Part model, mm, in its own coordinate system. A direction names the side the tool comes from. Round coordinates to 2 decimals unless told otherwise and drop trailing zeros. Loops run counter-clockwise (first coordinate to the right, second up) from the corner with the lowest first, then second, coordinate; pieces in that order, holes last.
Autodesk Inventor part; units mm, degrees
ref_plane "YZ Plane" through (0, 0, 0) normal (1, 0, 0) x (0, 1, 0)
ref_plane "XZ Plane" through (0, 0, 0) normal (0, 1, 0) x (-1, 0, 0)
ref_plane "XY Plane" through (0, 0, 0) normal (0, 0, 1) x (1, 0, 0)
sketch "Sketch1" plane through (0, 0, 0) normal (0, 1, 0) x (-1, 0, 0)
  line L0 (0.0381, -21.3061) -> (0.0381, -411.3061)
  line L1 (0.0381, -411.3061) -> (21.2513, -432.5193)
  line L2 (0.0381, -411.3061) -> (30.0381, -411.3061) construction
  line L3 (21.2513, -432.5193) -> (221.2513, -432.5193)
  line L4 (221.2513, -432.5193) -> (270.7487, -383.0218)
  line L5 (270.7487, -383.0218) -> (390.7487, -383.0218)
  line L6 (390.7487, -383.0218) -> (447.3173, -439.5904)
  line L7 (447.3173, -439.5904) -> (487.3173, -439.5904)
  line L8 (487.3173, -439.5904) -> (543.8858, -383.0218)
  line L9 (-53.2718, -216.3061) -> (592.6367, -216.3061) construction
  line L10 (0.0381, -21.3061) -> (21.2513, -0.0929)
  line L11 (21.2513, -0.0929) -> (221.2513, -0.0929)
  line L12 (221.2513, -0.0929) -> (270.7487, -49.5904)
  line L13 (270.7487, -49.5904) -> (390.7487, -49.5904)
  line L14 (390.7487, -49.5904) -> (447.3173, 6.9782)
  line L15 (447.3173, 6.9782) -> (487.3173, 6.9782)
  line L16 (487.3173, 6.9782) -> (543.8858, -49.5904)
  line L17 (543.8858, -383.0218) -> (543.8858, -49.5904)
  point P0 (0, 0)
  dimension "d0" = 390
  dimension "d1" = 30
  dimension "d2" = 45
  dimension "d3" = 70
  dimension "d4" = 135
  dimension "d5" = 200
  dimension "d6" = 120
  dimension "d7" = 80
  dimension "d8" = 135
  dimension "d9" = 226.066
  dimension "d10" = 21.2132
  dimension "d11" = 40
  dimension "d12" = 80
  dimension "d15" = 543.8478
extrude "Extrusion1" add sketch "Sketch1" along normal blind 200
sketch "Sketch2" plane through (-221.2513, 0, -0.0929) normal (0, 0, 1) x (1, 0, 0)
  line L0 (200, 0) -> (200, 200) construction
  line L1 (200, 50) -> (-356.3945, 50) construction
  line L2 (0, 0) -> (200, 0) construction
  line L3 (91.2132, 236.2215) -> (91.2132, -57.6692) construction
  line L4 (221.2132, 0) -> (221.2132, 200) construction
  point P0 (221.2513, 0)
  dimension "d18" = 50
  dimension "d19" = 130
sketch "Sketch3" plane through (-221.2513, 0, -0.0929) normal (0, 0, 1) x (1, 0, 0)
  line L0 (91.2132, 236.2215) -> (91.2132, -57.6692) construction
  line L1 (200, 50) -> (-356.3945, 50) construction
  circle A0 centre (91.2132, 50) radius 25
  point P0 (221.2513, 0)
  dimension "d20" = 50
properties part number "Frame"
1) Slice it at C-C, the plane x = -368. Give the cut face in (y, z).
Values:
outline: (0, -383.02) - (200, -383.02) - (200, -49.59) - (0, -49.59) - close
2) Mould opens along X. For faces 5 (the face through (-10.496, 98.6, -421.764)), 6 (the face through (-467, 99, -439.59)), 7 (the face through (-418.64, 98.6, -21.7)) say: released by +X, released by -X, zero draft, split by the parting line, or undercut.
Values:
face 5: released by +X
face 6: zero draft
face 7: undercut
3) Drop flat-ended pins along their axis: pin 1 Ø3 at (x, y) = (-288.5, 102.5) entering from +Z; pin 2 Ø10 at (x, y) = (-152.5, 49) entering from -Z; pin 3 Ø1 at (x, y) = (-249.5, 80) entering from -Z. Give the stop position or say it passes through.
Values:
pin 1: stops at z = -49.59
pin 2: stops at z = -432.52
pin 3: stops at z = -404.77
4) Tool access for faces 1 (the face through (-120, 99, -432.519)), 2 (the face through (-330, 99, -383.022)), 3 (the face through (-245.654, 98.6, -24.495)), 4 (the face through (-120, 99, -0.093)): list every direction of +Z, -Z, +X, -X, +Y, -Y with a clear straight run to the whole face (end or side of a thin tool).
Values:
face 1: -Z, +X, +Y, -Y
face 2: -Z, +Y, -Y
face 3: +Z, +Y, -Y
face 4: +Z, +X, +Y, -Y
5) Wall check: line 1 along Z through (x, y) = (-213.5, 108); line 2 along X through (y, z) = (144.5, -412.5); line 3 along Z through (x, y) = (-360, 170). Give the ranges that are in metal, low to high.
Values:
line 1: z = -432.52 to -0.09
line 2: x = -514.41 to -420.23, -241.27 to -1.23
line 3: z = -383.02 to -49.59
6) Slice it at A-A, the plane y = 115. Give the cut face in (x, z), then the cut area to 3 significant figures.
Values:
outline: (-543.89, -383.02) - (-487.32, -439.59) - (-447.32, -439.59) - (-390.75, -383.02) - (-270.75, -383.02) - (-221.25, -432.52) - (-21.25, -432.52) - (-0.04, -411.31) - (-0.04, -21.31) - (-21.25, -0.09) - (-221.25, -0.09) - (-270.75, -49.59) - (-390.75, -49.59) - (-447.32, 6.98) - (-487.32, 6.98) - (-543.89, -49.59) - close
area: 216,000 mm2
7) Slice it at B-B, the plane x = -58. Give the cut face in (y, z), then the cut area to 3 significant figures.
Values:
outline: (0, -432.52) - (200, -432.52) - (200, -0.09) - (0, -0.09) - close
area: 86,500 mm2
